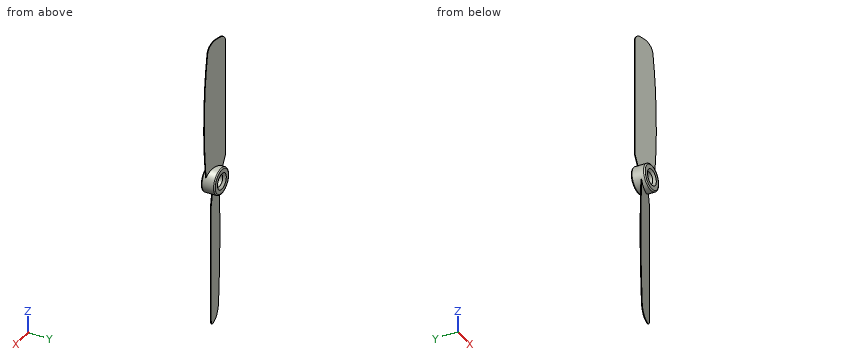
```python
from build123d import *

# Parameters (mm, degrees)
SKETCH1_R           = 5.75
BOSS_EXTRUDE1_DEPTH = 3
BOSS_EXTRUDE2_DEPTH = 0.15
CIRPATTERN1_COUNT   = 2
SKETCH4_R           = 2.5
CUT_EXTRUDE1_DEPTH  = 65.083925427
FILLET1_R           = 0.5
CHAMFER1_SIZE       = 1


with BuildPart() as part:
    # Sketch1 → Boss-Extrude1 (new, symmetric)
    with BuildSketch(Plane(origin=(0, 0, 0), x_dir=(1, 0, 0), z_dir=(0, 1, 0))):
        with Locations(Location((0, 0, 0), (0, 0, 270))):
            Circle(SKETCH1_R)
    extrude(amount=BOSS_EXTRUDE1_DEPTH, both=True)

    # Sketch3 → Boss-Extrude2 (add, symmetric)
    with BuildSketch(Plane(origin=(0, 0, 0), x_dir=(0.9743700647852351, -0.22495105434386545, 0), z_dir=(-0.22495105434386545, -0.9743700647852351, 0))):
        with BuildLine():
            Line((-3.946096789, 3.251337345), (-5.859151844, 8.548605509))
            Line((-5.859151844, 8.548605509), (-5.859151844, 60.5))
            ThreePointArc((-5.859151844, 60.5), (-4.980472188, 62.621320344), (-2.859151844, 63.5))
            Line((-2.859151844, 63.5), (-0.550434398, 63.5))
            ThreePointArc((-0.550434398, 63.5), (2.768651687, 62.239474236), (4.414220363, 59.093467024))
            add(Edge.make_bspline(
                [(5.295803115, 3.251337345), (6.928408565, 21.891598877), (6.634212966, 40.522095073), (4.414220363, 59.093467024)],
                knots=[0, 0, 0, 0, 0.926692818, 0.926692818, 0.926692818, 0.926692818], degree=3))
            add(Edge.make_bspline(
                [(5.295803115, 3.251337345), (0.674853163, 10.168892518), (-3.946096789, 3.251337345)],
                knots=[5.313367698, 5.313367698, 5.313367698, 7.253002917, 7.253002917, 7.253002917], degree=2, weights=[1, 0.565449973, 1]))
        make_face()
    boss_extrude2 = extrude(amount=BOSS_EXTRUDE2_DEPTH, both=True)

    # CirPattern1: Boss-Extrude2 ×2 about axis
    cirpattern1_axis = Axis((0, 3, 0), (0, 1, 0))
    for i in range(1, CIRPATTERN1_COUNT):
        add(boss_extrude2.rotate(cirpattern1_axis, i * 360 / CIRPATTERN1_COUNT))

    # Sketch4 → Cut-Extrude1 (cut, through all)
    with BuildSketch(Plane(origin=(0, 3, 0), x_dir=(1, 0, 0), z_dir=(0, 1, 0))):
        with Locations(Location((0, 0, 0), (0, 0, 270))):
            Circle(SKETCH4_R)
    extrude(amount=-CUT_EXTRUDE1_DEPTH, mode=Mode.SUBTRACT)

    # Fillet1
    fillet1_edges = [part.edges().sort_by_distance(p)[0] for p in [
        (0, -3, -5.75),
        (0, 3, -5.75),
    ]]
    fillet(fillet1_edges, radius=FILLET1_R)

    # Chamfer1
    chamfer1_edges = [part.edges().sort_by_distance(p)[0] for p in [
        (0, -3, -2.5),
        (0, 3, -2.5),
    ]]
    chamfer(chamfer1_edges, length=CHAMFER1_SIZE)


solid = part.part
```
Can you work these out from the model? Positions are in its coordinate system, mm. Coordinates: 2 decimals unless noted, no trailing zeros. Write each loop counter-clockwise with the first axis right and the second up, starting at its lowest first coordinate (ties: lowest second). Pieces come first, ordered by that corner, then holes. Notation, with made-up numbers: M -18,21.5 L -9,21.5 A19 ccw -9,44.5 Z; hole C -26,57 d1. An arc over 180 degrees is marked long. Answer as CSV lines item,"result".
Item 1: I'm going to push flat-ended pins straight in: P1, Ø3, axis at y = -1, z = 0.5, coming from the +X side; P2, Ø4, axis at x = 0, z = 0, coming from the +Y side. Where does each tip first touch, or does it pass through?
Geometry results:
P1,"stops at x = 5.75"
P2,"passes through"
Item 2: Please list where these lines run through material, in increasing order: line 1 along Z through (x, y) = (0, -2.25); line 2 along X through (y, z) = (1.2, 0); line 3 along Z through (x, y) = (0.25, 1.5).
Geometry results:
line 1,"z = -5.75 to -2.75, 2.75 to 5.75"
line 2,"x = -5.75 to -2.5, 2.5 to 5.75"
line 3,"z = -5.74 to -2.49, 2.49 to 5.74"
Item 3: Imagine slicing it at A-A on z = 0. List the corners of the cut face in (x, y) for me, plus the area to 3 significant figures.
Geometry results:
outline,"M -5.75,-2.5 A0.5 ccw -5.25,-3 L -3.5,-3 L -2.5,-2 L -2.5,2 L -3.5,3 L -5.25,3 A0.5 ccw -5.75,2.5 Z; M 2.5,-2 L 3.5,-3 L 5.25,-3 A0.5 ccw 5.75,-2.5 L 5.75,2.5 A0.5 ccw 5.25,3 L 3.5,3 L 2.5,2 Z"
area,"36.8 mm2"
